Autodesk Fusion 360 part; units mm, degrees
sketch "Esquisse1" plane through (0, 0, 0) normal (0, 0, 1) x (1, 0, 0)
  circle A0 centre (-55.5807, 0.978) radius 6.2
  circle A1 centre (-1.1807, 0.978) radius 4.2
  line L0 (-55.5807, 13.478) -> (-1.1807, 13.478)
  line L1 (-1.1807, 13.478) -> (-1.1807, -11.522) construction
  line L2 (-1.1807, -11.522) -> (-55.5807, -11.522)
  line L3 (-55.5807, -11.522) -> (-55.5807, 13.478) construction
  arc A2 (-55.5807, 13.478) -> (-55.5807, -11.522) centre (-55.5807, 0.978) ccw
  line L4 (9.7852, -5.022) -> (13.2852, -5.022)
  line L5 (13.2852, -5.022) -> (13.2852, 6.978)
  line L6 (13.2852, 6.978) -> (9.7852, 6.978)
  arc A3 (-1.1807, -11.522) -> (9.7852, -5.022) centre (-1.1807, 0.978) ccw
  arc A4 (9.7852, 6.978) -> (-1.1807, 13.478) centre (-1.1807, 0.978) ccw
  dimension "d1" = 54.4
  dimension "d2" = 12.4
  dimension "d3" = 8.4
  dimension "d4" = 25
  dimension "d5" = 12.5
  dimension "d7" = 12
  dimension "d8" = 3.5
extrude "Extrusion1" add sketch "Esquisse1" along normal blind 10
sketch "Esquisse2" plane through (0, 0, 10) normal (0, 0, 1) x (-1, 0, 0)
  circle A0 centre (55.5807, -0.978) radius 6.2
  circle A1 centre (1.1807, -0.978) radius 4.2
  arc A2 (1.1807, 11.522) -> (-9.7852, 5.022) centre (1.1807, -0.978) ccw
  line L0 (-9.7852, 5.022) -> (-13.2852, 5.022)
  line L1 (-13.2852, 5.022) -> (-13.2852, -6.978)
  line L2 (-13.2852, -6.978) -> (-9.7852, -6.978)
  arc A3 (-9.7852, -6.978) -> (1.1807, -13.478) centre (1.1807, -0.978) ccw
  line L3 (1.1807, -13.478) -> (55.5807, -13.478)
  arc A4 (55.5807, -13.478) -> (55.5807, 11.522) centre (55.5807, -0.978) ccw
  line L4 (55.5807, 11.522) -> (1.1807, 11.522)
  circle A5 centre (55.5807, -0.978) radius 7
  circle A6 centre (1.1807, -0.978) radius 5
  dimension "d11" = 14
  dimension "d12" = 10
extrude "Extrusion2" add sketch "Esquisse2" along normal blind 0.2 contours A5 | A6
ref_plane "Plan de construction2" through (10.2852, 0.978, 5) normal (1, 0, 0) x (0, 1, 0)
sketch "Esquisse3" plane through (10.2852, 0, 0) normal (1, 0, 0) x (0, 1, 0)
  line L0 (-5.022, 0) -> (6.978, 0)
  line L1 (6.978, 0) -> (6.978, 10)
  line L2 (6.978, 10) -> (-5.022, 10)
  line L3 (-5.022, 10) -> (-5.022, 0)
  line L4 (-2.022, 10) -> (3.978, 10)
  line L5 (3.978, 10) -> (3.978, 5)
  line L6 (3.978, 5) -> (-2.022, 5) construction
  line L7 (-2.022, 5) -> (-2.022, 10)
  line L8 (0.978, 5) -> (0.978, 1.9) construction
  line L9 (-2.022, 6.7321) -> (-2.022, 3.2679)
  line L10 (-2.022, 3.2679) -> (0.978, 1.5359)
  line L11 (0.978, 1.5359) -> (3.978, 3.2679)
  line L12 (3.978, 3.2679) -> (3.978, 6.7321)
  point P0 (0.978, 5)
  dimension "d15" = 3.1
  dimension "d16" = 5
  dimension "d17" = 6
  dimension "d18" = 12
  dimension "d19" = 3
extrude "Extrusion3" cut sketch "Esquisse3" against normal blind 2.4 contours L2 L4 L5 L7 L9 L10 L11 L12
hole "Perçage1" at (13.2852, 0.8569, 5) direction (-1, 0, 0) diameter 3.4 depth 11 tip angle 180
chamfer "Chanfrein1" distance 1 angle 45 16 edges at (5.1931, -9.7749, 10) (5.1931, 11.7309, 10) (-28.3807, 13.478, 10) (-68.0807, 0.978, 10) (-28.3807, -11.522, 10) (-28.3807, -11.522, 0) (-68.0807, 0.978, 0) (-28.3807, 13.478, 0) (5.1931, 11.7309, 0) (5.1931, -9.7749, 0) (11.5352, -5.022, 0) (11.5352, -5.022, 10) (13.2852, 0.978, 0) (13.2852, 0.978, 10) (11.5352, 6.978, 10) (11.5352, 6.978, 0)
chamfer "Chanfrein2" distance 1 angle 45 2 edges at (13.2852, 6.978, 5) (13.2852, -5.022, 5)
equation "d5 = d4 / 2"
equation "d19 = ( d18 - d17 ) / 2"
The listing builds one solid part. Answer for the finished solid, in the listing's coordinates (mm). A direction names the side the tool comes from. Round coordinates to 2 decimals unless told otherwise and drop trailing zeros. Loops run counter-clockwise (first coordinate to the right, second up) from the corner with the lowest first, then second, coordinate; pieces in that order, holes last.
Q1. Given pin 1 Ø1.9 at (x, z) = (9.5, 5.5) entering from +Y; pin 2 Ø4 at (x, z) = (1.5, 4) entering from -Y; pin 3 Ø1.2 at (x, z) = (8.5, 5) entering from -Y, each flat-ended and moving along its own axis, determine where each tip first touches the part or whether it passes through.
Q2. For a pull along Y with two mould halves and no side action, classify faces 1 (the face through (5.11, 11.78, 4.94)), 2 (the face through (10.285, 1, 7)), 3 (the face through (-67.25, 1.23, 0.17)), 4 (the face through (2, -2, 10.2)) as released by +Y, released by -Y, zero draft, split by the parting line, or undercut.
Q3. Section A-A, the plane z = 5 is taken. Determine the outline of the cut face in (x, y).
Q4. Find the intervals of material crossed by line 1 (Y direction, x = 12.05, z = 5); line 2 (X direction, y = 2.25, z = 7); line 3 (X direction, y = 3.5, z = 2), in increasing order.
Q5. Section B-B, the plane x = -27 is taken. Determine the outline of the cut face in (y, z).
Q6. Which of the six approach directions +Z, -Z, +X, -X, +Y, -Y give full straight-line access (tool end or side, diameter ignored) to faces 5 (the face through (11, 6.978, 5)), 6 (the face through (11.764, 0.346, 3.379)), 7 (the face through (9.1, -0.54, 2.41))?
Completed:
1. pin 1: stops at y = 8.82
1. pin 2: stops at y = -11.5
1. pin 3: stops at y = -7.61
2. face 1: released by +Y
2. face 2: undercut
2. face 3: split by the parting line
2. face 4: zero draft
3. outline: (-55.58, -11.52) - (-1.18, -11.52) arc R12.5 ccw to (9.79, -5.02) - (12.29, -5.02) - (13.29, -4.02) - (13.29, -0.84) - (10.29, -0.84) - (10.29, -2.02) - (7.89, -2.02) - (7.89, -0.84) - (2.6, -0.84) arc R4.2 cw (long way) to (2.71, 2.56) - (7.89, 2.56) - (7.89, 3.98) - (10.29, 3.98) - (10.29, 2.56) - (13.29, 2.56) - (13.29, 5.98) - (12.29, 6.98) - (9.79, 6.98) arc R12.5 ccw to (-1.18, 13.48) - (-55.58, 13.48) arc R12.5 ccw to start; hole circle Ø12.4 at (-55.58, 0.98)
4. line 1: y = -5.02 to -0.84, 2.56 to 6.98
4. line 2: x = -68.02 to -61.65, -49.51 to -5.18, 2.82 to 7.89, 10.29 to 13.29
4. line 3: x = -67.82 to -61.24, -49.92 to -4.54, 2.18 to 13.29
5. outline: (-11.52, 1) - (-10.52, 0) - (12.48, 0) - (13.48, 1) - (13.48, 9) - (12.48, 10) - (-10.52, 10) - (-11.52, 9) - close
6. face 5: +Z, -Z, +X, +Y
6. face 6: +X
6. face 7: +Z
